CAD build for the part. Positions are in the model's coordinates, mm. Give positions to 0.01 mm unless a question says otherwise; leave off trailing zeros. Loops run counter-clockwise (first coordinate to the right, second up) from the corner with the lowest first, then second, coordinate; pieces in that order, holes last.
Autodesk Inventor part; units mm, degrees
ref_plane "rod_cp_XY" through (0, 0, 0) normal (1, 0, 0) x (0, 0, -1)
ref_plane "rod_cp_YZ" through (0, 0, 0) normal (0, 0, -1) x (0, 1, 0)
ref_plane "rod_cp_ZX" through (0, 0, 0) normal (0, 1, 0) x (1, 0, 0)
sketch "Sketch_1" plane through (0, 0, 0) normal (0, 0, 1) x (1, 0, 0)
  line L0 (111.9124, 0) -> (0, 0)
  line L1 (0, 0) -> (0, 3.175)
  line L2 (0, 3.175) -> (91.2876, 3.175)
  line L3 (91.2876, 3.175) -> (91.2876, 9.6203)
  line L4 (91.2876, 9.6203) -> (111.9124, 9.6203)
  line L5 (111.9124, 9.6203) -> (111.9124, 0)
  line L6 (111.9124, 0) -> (0, 0)
revolve "Revolution1" add sketch "Sketch_1" angle 360 about axis through (111.9124, 0, 0) along (1, 0, 0)
sketch "Sketch_3" plane through (0, 0, 0) normal (0, 0, 1) x (1, 0, 0)
  line L0 (0, 0) -> (-12.7, 0)
  line L1 (-12.7, 0) -> (-12.7, 2.634)
  line L2 (-12.7, 2.634) -> (-12.159, 3.175)
  line L3 (-12.159, 3.175) -> (0, 3.175)
  line L4 (0, 3.175) -> (0, 0)
  line L5 (0, 0) -> (-12.7, 0)
revolve "Revolution2" add sketch "Sketch_3" angle 360 about axis through (0, 0, 0) along (1, 0, 0)
sketch "Sketch_6" plane through (0, 0, 0) normal (0, 0, 1) x (1, 0, 0)
  line L0 (203.2, 0) -> (111.9124, 0)
  line L1 (111.9124, 0) -> (111.9124, 3.175)
  line L2 (111.9124, 3.175) -> (203.2, 3.175)
  line L3 (203.2, 3.175) -> (203.2, 0)
  line L4 (203.2, 0) -> (111.9124, 0)
revolve "Revolution3" add sketch "Sketch_6" angle 360 about axis through (203.2, 0, 0) along (1, 0, 0)
sketch "Sketch_7" plane through (0, 0, 0) normal (0, 0, 1) x (1, 0, 0)
  line L0 (215.9, 0) -> (203.2, 0)
  line L1 (203.2, 0) -> (203.2, 3.175)
  line L2 (203.2, 3.175) -> (215.359, 3.175)
  line L3 (215.359, 3.175) -> (215.9, 2.634)
  line L4 (215.9, 2.634) -> (215.9, 0)
  line L5 (215.9, 0) -> (203.2, 0)
revolve "Revolution4" add sketch "Sketch_7" angle 360 about axis through (215.9, 0, 0) along (1, 0, 0)
sketch "Sketch_30" plane through (0, 0, 0) normal (0, 0, 1) x (1, 0, 0)
  line L0 (0, 0) -> (-0.254, 0)
  line L1 (-0.254, 3.429) -> (-0.254, 2.921)
  line L2 (-0.254, 2.921) -> (0, 2.921)
  line L3 (0, 2.921) -> (0, 3.429)
  line L4 (0, 3.429) -> (-0.254, 3.429)
revolve "Revolution5" cut sketch "Sketch_30" angle 360 about axis through (0, 0, 0) along (1, 0, 0)
sketch "Sketch_40" plane through (0, 0, 0) normal (0, 0, 1) x (1, 0, 0)
  line L0 (203.454, 0) -> (203.2, 0)
  line L1 (203.2, 3.429) -> (203.2, 2.921)
  line L2 (203.2, 2.921) -> (203.454, 2.921)
  line L3 (203.454, 2.921) -> (203.454, 3.429)
  line L4 (203.454, 3.429) -> (203.2, 3.429)
revolve "Revolution6" cut sketch "Sketch_40" angle 360 about axis through (203.454, 0, 0) along (1, 0, 0)
ref_plane "rod_cp_XY" through (0, 0, 0) normal (1, 0, 0) x (0, 0, -1)
ref_plane "rod_cp_YZ" through (0, 0, 0) normal (0, 0, -1) x (0, 1, 0)
ref_plane "rod_cp_ZX" through (0, 0, 0) normal (0, 1, 0) x (1, 0, 0)
ref_plane "to_rod_clevis_XY" through (-12.7, 0, 0) normal (1, 0, 0) x (0, 0, -1)
ref_plane "to_rod_clevis_YZ" through (-12.7, 0, 0) normal (0, 0, -1) x (0, 1, 0)
ref_plane "to_rod_clevis_ZX" through (-12.7, 0, 0) normal (0, 1, 0) x (1, 0, 0)
ref_plane "rl2_XY" through (0, 0, 0) normal (1, 0, 0) x (0, 0, -1)
ref_plane "rl2_YZ" through (0, 0, 0) normal (0, 0, -1) x (0, 1, 0)
ref_plane "rl2_ZX" through (0, 0, 0) normal (0, 1, 0) x (1, 0, 0)
ref_plane "rl1_XY" through (-12.7, 0, 0) normal (1, 0, 0) x (0, 0, -1)
ref_plane "rl1_YZ" through (-12.7, 0, 0) normal (0, 0, -1) x (0, 1, 0)
ref_plane "rl1_ZX" through (-12.7, 0, 0) normal (0, 1, 0) x (1, 0, 0)
ref_plane "rl1_der_XY" through (215.9, 0, 0) normal (1, 0, 0) x (0, 0, -1)
ref_plane "rl1_der_YZ" through (215.9, 0, 0) normal (0, 0, -1) x (0, 1, 0)
ref_plane "rl1_der_ZX" through (215.9, 0, 0) normal (0, 1, 0) x (1, 0, 0)
ref_plane "rl2_der_XY" through (203.2, 0, 0) normal (1, 0, 0) x (0, 0, -1)
ref_plane "rl2_der_YZ" through (203.2, 0, 0) normal (0, 0, -1) x (0, 1, 0)
ref_plane "rl2_der_ZX" through (203.2, 0, 0) normal (0, 1, 0) x (1, 0, 0)
ref_plane "thd1_XY" through (-12.7, 3.175, 0) normal (1, 0, 0) x (0, 0, -1)
ref_plane "thd1_YZ" through (-12.7, 3.175, 0) normal (0, 0, -1) x (0, 1, 0)
ref_plane "thd1_ZX" through (-12.7, 3.175, 0) normal (0, 1, 0) x (1, 0, 0)
ref_plane "thd2_XY" through (-12.7, -3.175, 0) normal (1, 0, 0) x (0, 0, -1)
ref_plane "thd2_YZ" through (-12.7, -3.175, 0) normal (0, 0, -1) x (0, 1, 0)
ref_plane "thd2_ZX" through (-12.7, -3.175, 0) normal (0, 1, 0) x (1, 0, 0)
ref_plane "dia1_XY" through (0, 3.175, 0) normal (1, 0, 0) x (0, 0, -1)
ref_plane "dia1_YZ" through (0, 3.175, 0) normal (0, 0, -1) x (0, 1, 0)
ref_plane "dia1_ZX" through (0, 3.175, 0) normal (0, 1, 0) x (1, 0, 0)
ref_plane "dia2_XY" through (0, -3.175, 0) normal (1, 0, 0) x (0, 0, -1)
ref_plane "dia2_YZ" through (0, -3.175, 0) normal (0, 0, -1) x (0, 1, 0)
ref_plane "dia2_ZX" through (0, -3.175, 0) normal (0, 1, 0) x (1, 0, 0)
ref_plane "stroke1_XY" through (0, 0, 0) normal (1, 0, 0) x (0, 0, -1)
ref_plane "stroke1_YZ" through (0, 0, 0) normal (0, 0, -1) x (0, 1, 0)
ref_plane "stroke1_ZX" through (0, 0, 0) normal (0, 1, 0) x (1, 0, 0)
ref_plane "dia12_XY" through (0, 0, 10.9537) normal (1, 0, 0) x (0, 0, -1)
ref_plane "dia12_YZ" through (0, 0, 10.9537) normal (0, 0, -1) x (0, 1, 0)
ref_plane "dia12_ZX" through (0, 0, 10.9537) normal (0, 1, 0) x (1, 0, 0)
ref_plane "dia22_XY" through (0, 0, -10.9537) normal (1, 0, 0) x (0, 0, -1)
ref_plane "dia22_YZ" through (0, 0, -10.9537) normal (0, 0, -1) x (0, 1, 0)
ref_plane "dia22_ZX" through (0, 0, -10.9537) normal (0, 1, 0) x (1, 0, 0)
properties part number "042-DXDE0_rod"
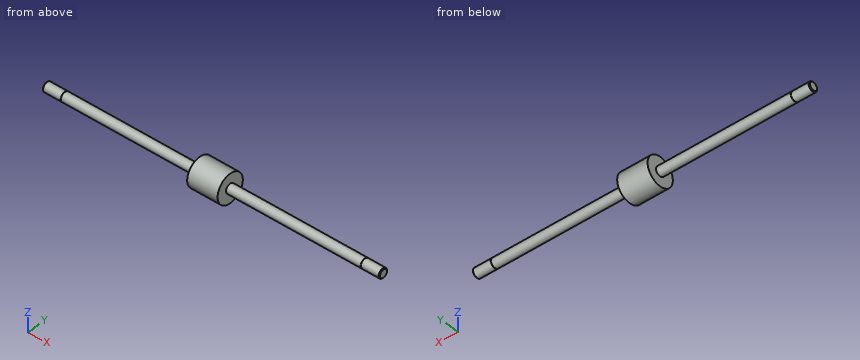
1. Saw through at C-C, the plane x = 63. List the corners of the cut face in (y, z) (3 decimals).
Responses:
outline: circle Ø6.35 at (0, 0)
2. Drop flat-ended pins along their axis: pin 1 (5 mm diameter, centred on y = 7.5, z = -6, fed in from +X); pin 2 (2 mm diameter, centred on y = 7.5, z = 0, fed in from -X); pin 3 (10 mm diameter, centred on x = 120, z = 6, fed in from -Y); pin 4 (9.5 mm diameter, centred on y = 0, z = -4.5, fed in from -X). Give the stop position or say it passes through.
Responses:
pin 1: stops at x = 111.91
pin 2: stops at x = 91.29
pin 3: stops at y = -3.01
pin 4: stops at x = -12.7
3. Probe line 1 along X through (y, z) = (6.5, -3.25); line 2 along Z through (x, y) = (59, -0.5); line 3 along Y through (x, z) = (108, 4.75). List the from-to ranges inside material, lowest first.
Responses:
line 1: x = 91.29 to 111.91
line 2: z = -3.14 to 3.14
line 3: y = -8.37 to 8.37
